Could you check a few things on this model? Use its own coordinates, in mm. Coordinates: 2 decimals unless noted, no trailing zeros. Loops run counter-clockwise (first coordinate to the right, second up) from the corner with the lowest first, then second, coordinate; pieces in that order, holes last.
1) Imagine slicing it at D-D on y = -8.5. Please give me the cut outline in (x, z).
2) Imagine slicing it at A-A on x = 0. Please give me the cut outline in (y, z), plus the area to 3 significant figures.
3) Imagine slicing it at C-C on z = 46. Please give me the cut outline in (x, y).
4) Imagine slicing it at B-B on y = 0. Please give me the cut outline in (x, z), plus the area to 3 significant figures.
5) If I drill on line 1 along Z through (x, y) = (-9, 5.5); line 2 along Y through (x, z) = (0, 109); line 3 along Z through (x, y) = (-14, 9), over which ranges is the centre line in solid material (lowest first)?
6) Will these pins go through, and if not, where does the flat tip stop? P1, Ø1, axis at x = 14, z = 24.5, coming from the -Y side; P2, Ø1, axis at y = -9.5, z = 50.5, coming from the -X side; P3, Ø8, axis at x = -15, z = 73.5, coming from the +Y side.
```python
from build123d import *

# Parameters (mm, degrees)
PAD_DEPTH       = 120
SKETCH001_R     = 6
POCKET_DEPTH    = 40
SKETCH002_R     = 1.7
POCKET001_DEPTH = 14
SKETCH003_R     = 3
POCKET002_DEPTH = 3
SKETCH004_R     = 2.2
POCKET003_DEPTH = 5
FILLET_R        = 5


with BuildPart() as part:
    # Sketch → Pad (new body)
    with BuildSketch(Plane.XY):
        Polygon((10.25, -17.7535207776), (20.5, 0), (10.25, 17.7535207776), (-10.25, 17.7535207776), (-20.5, 0), (-10.25, -17.7535207776), align=None)
    extrude(amount=PAD_DEPTH)

    # Sketch001 (on Face8 of Pad) → Pocket (cut)
    with BuildSketch(Plane.XY.offset(120)):
        Circle(SKETCH001_R)
    extrude(amount=-POCKET_DEPTH, mode=Mode.SUBTRACT)

    # Sketch002 (on Face8 of Pocket) → Pocket001 (cut)
    with BuildSketch(Plane(origin=(-15.375, 8.8767603888, 0), x_dir=(-0.5, -0.8660254038, 0), z_dir=(-0.8660254038, 0.5, 0))):
        with Locations((-3.77921e-05, 109.999999997)):
            Circle(SKETCH002_R)
        with Locations((0, 97.5)):
            Circle(SKETCH002_R)
        with Locations((-0.0004273495, 85)):
            Circle(SKETCH002_R)
    extrude(amount=-POCKET001_DEPTH, mode=Mode.SUBTRACT)

    # Sketch003 (on Face8 of Pocket001) → Pocket002 (cut)
    with BuildSketch(Plane(origin=(-15.375, 8.8767603888, 0), x_dir=(-0.5, -0.8660254038, 0), z_dir=(-0.8660254038, 0.5, 0))):
        with Locations((-0.0004273495, 85)):
            Circle(SKETCH003_R)
        with Locations((0, 97.5)):
            Circle(SKETCH003_R)
        with Locations((-3.77921e-05, 109.999999997)):
            Circle(SKETCH003_R)
    extrude(amount=-POCKET002_DEPTH, mode=Mode.SUBTRACT)

    # Sketch004 (on Face18 of Pocket002) → Pocket003 (cut)
    with BuildSketch(Plane(origin=(-12.7769237886, 7.3767603888, 0), x_dir=(-0.5, -0.8660254038, 0), z_dir=(-0.8660254038, 0.5, 0))):
        with Locations((-0.0004273495, 85)):
            Circle(SKETCH004_R)
        with Locations((-3.77921e-05, 109.999999997)):
            Circle(SKETCH004_R)
        with Locations((0, 97.5)):
            Circle(SKETCH004_R)
    extrude(amount=-POCKET003_DEPTH, mode=Mode.SUBTRACT)

    # Fillet
    fillet_edges = [part.edges().sort_by_distance(p)[0] for p in [
        (20.5, 0, 60),
        (-20.5, 0, 60),
        (10.25, -17.753521, 60),
        (-10.25, -17.753521, 60),
        (-10.25, 17.753521, 60),
        (10.25, 17.753521, 60),
    ]]
    fillet(fillet_edges, radius=FILLET_R)


solid = part.part
```
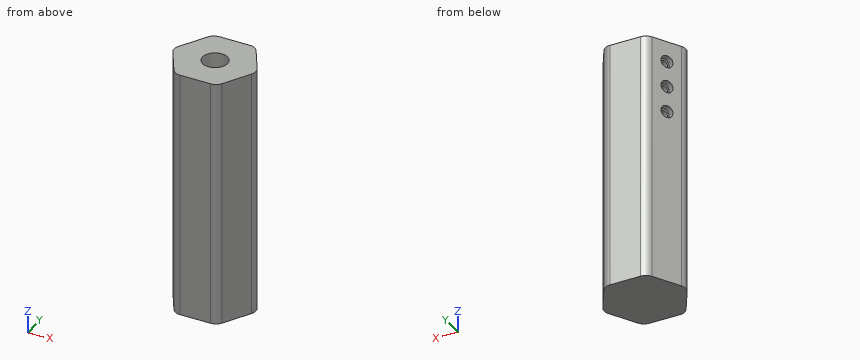
Filled in:
1. outline: (-15.59, 0) - (15.59, 0) - (15.59, 120) - (-15.59, 120) - close
2. outline: (-17.75, 0) - (17.75, 0) - (17.75, 120) - (6, 120) - (6, 80) - (-6, 80) - (-6, 120) - (-17.75, 120) - close
2. area: 3,780 mm2
3. outline: (-19.06, -2.5) - (-11.69, -15.25) arc R5 ccw to (-7.36, -17.75) - (7.36, -17.75) arc R5 ccw to (11.69, -15.25) - (19.06, -2.5) arc R5 ccw to (19.06, 2.5) - (11.69, 15.25) arc R5 ccw to (7.36, 17.75) - (-7.36, 17.75) arc R5 ccw to (-11.69, 15.25) - (-19.06, 2.5) arc R5 ccw to start
4. outline: (-19.73, 0) - (19.73, 0) - (19.73, 120) - (6, 120) - (6, 80) - (-6, 80) - (-6, 120) - (-19.73, 120) - close
4. area: 4,250 mm2
5. line 1: z = 0 to 82.82, 87.18 to 95.32, 99.68 to 107.82, 112.18 to 120
5. line 2: y = -17.75 to -6, 6 to 17.75
5. line 3: z = 0 to 82.11, 87.89 to 94.61, 100.39 to 107.11, 112.89 to 120
6. P1: stops at y = -12.12
6. P2: stops at x = -15.3
6. P3: stops at y = 16.18
